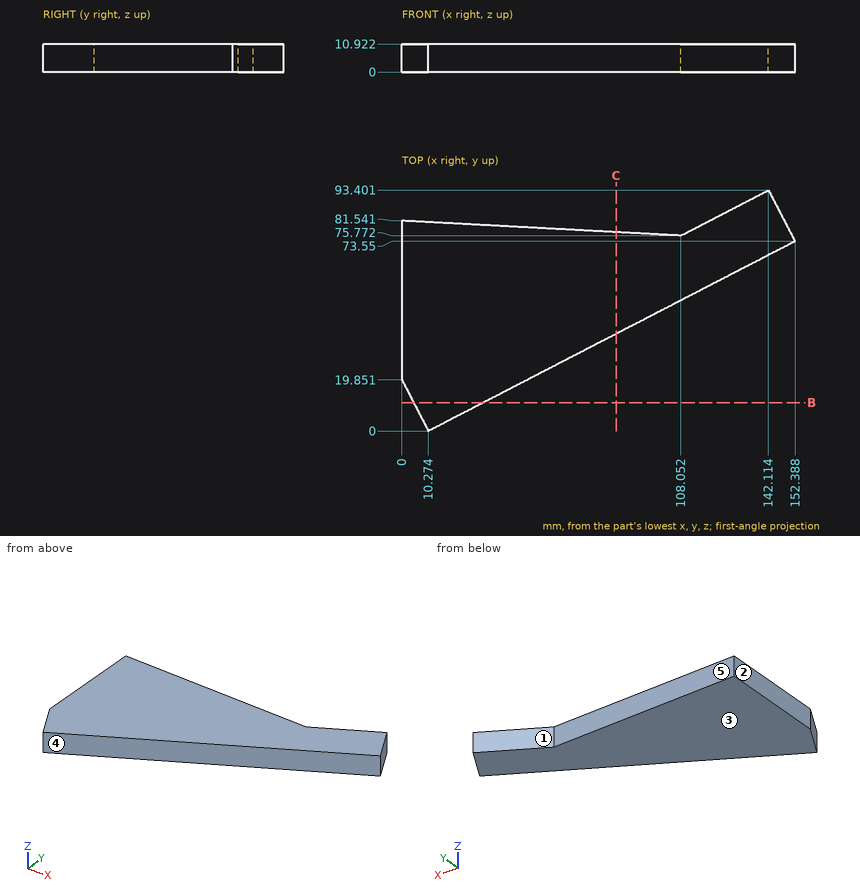
Study the drawing (mm; zero at the part's minimum x, y, z) and answer. A direction names the side the tool comes from. Coordinates: 2 decimals unless noted, no trailing zeros. Write each loop counter-clockwise with the first axis right and the second up, starting at its lowest first coordinate (ties: lowest second). Pieces come first, ordered by that corner, then holes. Notation, with made-up numbers: (71, 18.25) - (75, 18.25) arc R3 ccw to (75, 22.25) - close; hole circle Ø2 at (-32, 15.25). An arc over 180 degrees is marked (long way). One line per item, written item: value.
1) Find section B-B (y = 11). Give the vertices of the cut face in (x, z).
Geometry check:
outline: (4.58, 0) - (31.53, 0) - (31.53, 10.92) - (4.58, 10.92) - close
2) Consider line 1 along X through (y, z) = (74, 2.25) (1 decimal); line 2 along X through (y, z) = (23.5, 9) (1 decimal); line 3 along Y through (x, z) = (88, 2.5) (1 decimal). Determine where each line is inside the solid, lowest interval first. Write a range as from..to.
Geometry check:
line 1: x = 0..152.2
line 2: x = 0..55.7
line 3: y = 40.2..76.8
3) For a pull along X with two mould halves and no side action, classify the marked faces 1, 2 and 3 as pulls with the +X half, pulls with the -X half, needs draft (parallel to the pull), parting line crosses it, or undercut.
Geometry check:
face 1: undercut
face 2: pulls with the -X half
face 3: needs draft
4) A tool of negligible diameter and unlimited length cuts with its end or side. For the marked faces 4 and 5, from which of +Z, -Z, +X, -X, +Y, -Y can it reach the whole face along a straight path? Write none if from no direction.
Geometry check:
face 4: +Z, -Z, +X, -Y
face 5: +Z, -Z, +Y
5) Each of these flat-tipped pins is pushed along its axis until it touches: pin 1 Ø2 at (y, z) = (39, 5.5) entering from +X (1 decimal); pin 2 Ø5 at (y, z) = (44, 9) entering from -X; pin 3 Ø2 at (y, z) = (16, 1.5) entering from +X; pin 4 Ø5 at (y, z) = (11, 2.5) entering from +X. Where does it stop, or does it pass through?
Geometry check:
pin 1: stops at x = 87.6
pin 2: stops at x = 0
pin 3: stops at x = 43.12
pin 4: stops at x = 36.36
6) Find section C-C (x = 83). Give the vertices of the cut face in (y, z).
Geometry check:
outline: (37.64, 0) - (77.11, 0) - (77.11, 10.92) - (37.64, 10.92) - close
